Autodesk Inventor part; units mm, degrees
ref_plane "YZ Plane" through (0, 0, 0) normal (1, 0, 0) x (0, 1, 0)
ref_plane "XZ Plane" through (0, 0, 0) normal (0, 1, 0) x (-1, 0, 0)
ref_plane "XY Plane" through (0, 0, 0) normal (0, 0, 1) x (1, 0, 0)
sketch "Sketch1" plane through (0, 0, 0) normal (0, 0, 1) x (1, 0, 0)
  line L0 (0, 0) -> (41.6, 0)
  line L1 (41.6, 0) -> (41.6, 20)
  line L2 (41.6, 20) -> (0, 20)
  line L3 (0, 20) -> (0, 0)
  dimension "d0" = 41.6
  dimension "d1" = 20
extrude "Extrusion1" add sketch "Sketch1" along normal blind 10
sketch "Sketch3" plane through (0, 0, 10) normal (0, 0, 1) x (1, 0, 0)
  line L0 (0, 20) -> (5, 20)
  line L1 (5, 20) -> (5, 10)
  line L2 (5, 10) -> (0, 10)
  line L3 (0, 10) -> (0, 20)
  line L4 (41.6, 20) -> (36.6, 20)
  line L5 (36.6, 20) -> (36.6, 10)
  line L6 (36.6, 10) -> (41.6, 10)
  line L7 (41.6, 10) -> (41.6, 20)
  dimension "d7" = 5
  dimension "d8" = 5
  dimension "d9" = 10
extrude "Extrusion2" cut sketch "Sketch3" against normal through all
sketch "Sketch4" plane through (0, 0, 10) normal (0, 0, 1) x (1, 0, 0)
  line L0 (36.6, 20) -> (5, 20)
  line L1 (5, 20) -> (5, 10)
  line L2 (10, 20) -> (31.6, 20)
  line L3 (31.6, 20) -> (31.6, 10)
  line L4 (31.6, 10) -> (10, 10)
  line L5 (10, 10) -> (10, 20)
  dimension "d12" = 21.6
  dimension "d13" = 10
  dimension "d14" = 5
extrude "Extrusion3" cut sketch "Sketch4" against normal through all
fillet "Fillet1" radius 5 6 edges at (20.8, 0, 0) (20.8, 0, 10) (34.1, 20, 10) (34.1, 20, 0) (7.5, 20, 0) (7.5, 20, 10)
sketch "Sketch5" plane through (10, 10, 10) normal (0, 1, 0) x (1, 0, 0)
  line L0 (0, 10) -> (21.6, 10)
  line L1 (0, 0) -> (0, 10)
  line L2 (21.6, 0) -> (0, 0)
  line L3 (21.6, 0) -> (21.6, 10)
  point P0 (-10, 10)
extrude "Extrusion4" cut sketch "Sketch5" against normal blind 5
sketch "Sketch6" plane through (36.6, 10, 10) normal (0, 1, 0) x (1, 0, 0)
  line L0 (0, 10) -> (5, 10)
  line L1 (0, 0) -> (0, 10)
  line L2 (5, 0) -> (0, 0)
  line L3 (5, 10) -> (5, 0)
  point P0 (-36.6, 10)
extrude "Extrusion5" cut sketch "Sketch6" against normal blind 5
sketch "Sketch7" plane through (0, 10, 10) normal (0, 1, 0) x (1, 0, 0)
  line L0 (0, 10) -> (5, 10)
  line L1 (0, 0) -> (0, 10)
  line L2 (5, 0) -> (0, 0)
  line L3 (5, 0) -> (5, 10)
extrude "Extrusion6" cut sketch "Sketch7" against normal blind 5
sketch "Sketch8" plane through (5, 15, 5) normal (-1, 0, 0) x (0, 0, 1)
  arc A0 (5, 0) -> (-5, 0) centre (0, 0) ccw
  line L0 (-5, -10) -> (-5, 0)
  line L1 (-5, -10) -> (5, -10)
  line L2 (5, 0) -> (5, -10)
  point P0 (-5, -15)
extrude "Extrusion7" cut sketch "Sketch8" against normal blind 0.5
sketch "Sketch9" plane through (36.6, 15, 5) normal (1, 0, 0) x (0, 0, -1)
  arc A0 (5, 0) -> (-5, 0) centre (0, 0) ccw
  line L0 (-5, -10) -> (-5, 0)
  line L1 (-5, -10) -> (5, -10)
  line L2 (5, 0) -> (5, -10)
  point P0 (5, -15)
extrude "Extrusion8" cut sketch "Sketch9" against normal blind 0.5
sketch "Sketch10" plane through (36.1, 15, 5) normal (1, 0, 0) x (0, 0, -1)
  arc A0 (5, 0) -> (-5, 0) centre (0, 0) ccw
  circle A1 centre (0, 0) radius 2
  point P0 (5, -15)
  dimension "d28" = 4
extrude "Extrusion9" cut sketch "Sketch10" against normal through all
sketch "Sketch11" plane through (31.6, 15, 5) normal (-1, 0, 0) x (0, 0, 1)
  circle A0 centre (0, 0) radius 2
  arc A1 (5, 0) -> (-5, 0) centre (0, 0) ccw
  line L0 (5, 0) -> (5, -10)
  line L1 (-3.7, 1.5199) -> (-3.7, -1.5199)
  line L2 (3.7, 1.5199) -> (3.7, -1.5199)
  arc A2 (-3.7, -1.5199) -> (3.7, -1.5199) centre (0, 0) ccw
  arc A3 (3.7, 1.5199) -> (-3.7, 1.5199) centre (0, 0) ccw
  point P0 (-5, -15)
  dimension "d33" = 3.7
extrude "Extrusion10" cut sketch "Sketch11" against normal blind 1
sketch "Sketch12" plane through (10, 15, 5) normal (1, 0, 0) x (0, 0, -1)
  circle A0 centre (0, 0) radius 2
  arc A1 (5, 0) -> (-5, 0) centre (0, 0) ccw
  line L0 (5, 0) -> (5, -10)
  line L1 (3.7, 1.5199) -> (3.7, -1.5199)
  line L2 (-3.7, 1.5199) -> (-3.7, -1.5199)
  arc A2 (-3.7, -1.5199) -> (3.7, -1.5199) centre (0, 0) ccw
  arc A3 (3.7, 1.5199) -> (-3.7, 1.5199) centre (0, 0) ccw
  point P0 (5, -15)
  dimension "d37" = 3.7
extrude "Extrusion11" cut sketch "Sketch12" against normal blind 1
properties part number "Sliide"
Part model, mm, in its own coordinate system. A direction names the side the tool comes from. Round coordinates to 2 decimals unless told otherwise and drop trailing zeros. Loops run counter-clockwise (first coordinate to the right, second up) from the corner with the lowest first, then second, coordinate; pieces in that order, holes last. Notation, with made-up numbers: (-10, -35.75) -> (-5, -35.75) arc R15 ccw to (-5, -22.75) -> close; hole circle Ø5 at (-26, -8.5). An arc over 180 degrees is marked (long way). Use one line per item in the form item = value. Start each with the question number.
Item 1: Two-plate mould, pull along X, no slides. Class faces 4 (the cylindrical face through (34, 17, 5)), 5 (the flat face through (9.5, 15, 1.3)), 6 (the flat face through (0, 3, 5)): released by +X, released by -X, zero draft, split by the parting line, or undercut.
Item 2: Drill centre lines: line 1 along X through (y, z) = (10.25, 7.5); line 2 along X through (y, z) = (11.5, 6.25). Where is each one in solid material? Low to high.
Item 3: Band-saw the part on D-D (z = 6). List the corners of the cut face in (x, y).
Item 4: Band-saw the part on C-C (y = 18). List the corners of the cut face in (x, z), plus the area to 3 significant figures.
Item 5: Band-saw the part on B-B (z = 3.5). List the corners of the cut face in (x, y), plus the area to 3 significant figures.
Item 6: Drop flat-ended pins along their axis: pin 1 Ø2 at (y, z) = (11, 6.5) entering from +X; pin 2 Ø4 at (y, z) = (13, 7.5) entering from -X; pin 3 Ø3 at (x, z) = (20, 3.5) entering from +Y. Give the stop position or say it passes through.
Item 7: Tool access for faces 1 (the flat face through (39, 5, 5)), 2 (the cylindrical face through (32, 19, 5)), 3 (the cylindrical face through (34, 19, 2)): list every direction of +Z, -Z, +X, -X, +Y, -Y with a clear straight run to the whole face (end or side of a thin tool).
Data:
q1.face_4 = zero draft
q1.face_5 = undercut
q1.face_6 = released by -X
q2.line_1 = 5.5 to 10, 31.6 to 36.1
q2.line_2 = 5.5 to 9, 32.6 to 36.1
q3.outline = (0, 0.1) -> (41.6, 0.1) -> (41.6, 5) -> (36.1, 5) -> (36.1, 13.27) -> (32.6, 13.27) -> (32.6, 11.13) -> (31.6, 11.13) -> (31.6, 5) -> (10, 5) -> (10, 11.13) -> (9, 11.13) -> (9, 13.27) -> (5.5, 13.27) -> (5.5, 5) -> (0, 5) -> close; (5.5, 16.73) -> (9, 16.73) -> (9, 18.87) -> (10, 18.87) -> (10, 19.9) -> (5.5, 19.9) -> close; (31.6, 18.87) -> (32.6, 18.87) -> (32.6, 16.73) -> (36.1, 16.73) -> (36.1, 19.9) -> (31.6, 19.9) -> close
q4.outline = (5.5, 1) -> (10, 1) -> (10, 2.35) -> (9, 2.35) -> (9, 7.65) -> (10, 7.65) -> (10, 9) -> (5.5, 9) -> close; (31.6, 1) -> (36.1, 1) -> (36.1, 9) -> (31.6, 9) -> (31.6, 7.65) -> (32.6, 7.65) -> (32.6, 2.35) -> (31.6, 2.35) -> close
q4.area = 61.4 mm^2
q5.outline = (0, 0.23) -> (41.6, 0.23) -> (41.6, 5) -> (36.1, 5) -> (36.1, 13.68) -> (32.6, 13.68) -> (32.6, 11.29) -> (31.6, 11.29) -> (31.6, 5) -> (10, 5) -> (10, 11.29) -> (9, 11.29) -> (9, 13.68) -> (5.5, 13.68) -> (5.5, 5) -> (0, 5) -> close; (5.5, 16.32) -> (9, 16.32) -> (9, 18.71) -> (10, 18.71) -> (10, 19.77) -> (5.5, 19.77) -> close; (31.6, 18.71) -> (32.6, 18.71) -> (32.6, 16.32) -> (36.1, 16.32) -> (36.1, 19.77) -> (31.6, 19.77) -> close
q5.area = 298 mm^2
q6.pin_1 = 36.1
q6.pin_2 = 5.5
q6.pin_3 = 5
q7.face_1 = +Z, -Z, +X, +Y
q7.face_2 = none
q7.face_3 = -Z, +X, -X, +Y
